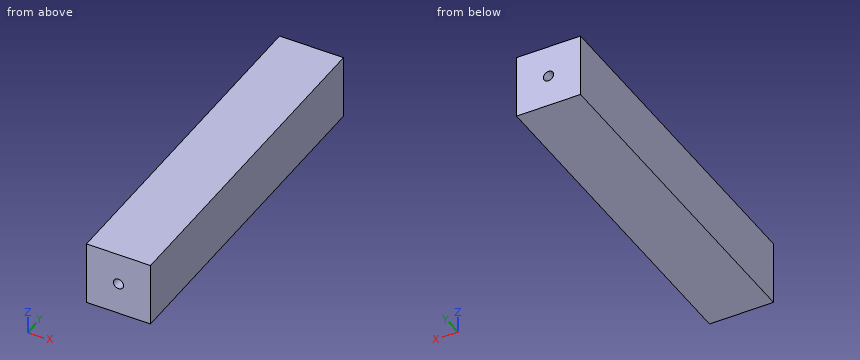
from build123d import *

# Parameters (mm, degrees)
F1_DEPTH = 250
F2_W     = 50
F2_H     = 50
F2_R     = 4
F3_DEPTH = 9.5
F4_W     = 50
F4_H     = 50
F4_R     = 4
F5_DEPTH = 9.5


with BuildPart() as f1:
    # F0 (on Front) → F1 (new body)
    with BuildSketch(Plane.XZ):
        Polygon((25, -25), (25, 0), (25, 25), (-25, 25), (-25, -25), align=None)
        Polygon((20, -20), (0, -20), (-20, -20), (-20, 20), (20, 20), align=None, mode=Mode.SUBTRACT)
    extrude(amount=F1_DEPTH)

    # F2 (on face) → F3 (join)
    with BuildSketch(Plane.XZ.offset(250)):
        Rectangle(F2_W, F2_H)
        Circle(F2_R, mode=Mode.SUBTRACT)
    extrude(amount=F3_DEPTH)

    # F4 (on face) → F5 (join)
    with BuildSketch(Plane.XZ):
        Rectangle(F4_W, F4_H)
        Circle(F4_R, mode=Mode.SUBTRACT)
    extrude(amount=-F5_DEPTH)


solid = f1.part
Here's how the part is built. I have some questions about the finished solid (model axes, mm). Give positions to 0.01 mm unless a question says otherwise; leave off trailing zeros. Order: outer loops, then holes, each group sorted by start corner. A loop starts at its lowest first (then second) coordinate and runs counter-clockwise, first axis right, second up. Notation, with made-up numbers: (-12.5, 49) -> (21.5, 49) arc R15 ccw to (21.5, 65) -> close; hole circle Ø10 at (60, -9). An arc over 180 degrees is marked (long way). Use a Markdown table: item, result. Add a question column.
Item 1: Imagine slicing it at A-A on x = 0. Please give me the cut outline in (y, z).
Item 2: I need wall thicknesses on line 1 (Z direction, x = -15, y = -199.5); line 2 (Y direction, x = 2, z = -17). Which ranges of each line are inside material? Lowest first, please.
Item 3: Imagine slicing it at B-B on z = -8. Please give me the cut outline in (x, y).
Item 4: Imagine slicing it at C-C on y = -66. Please give me the cut outline in (x, z).
Data:
| question | item | result |
|---|---|---|
| 1 | outline | (-259.5, -25) -> (9.5, -25) -> (9.5, -4) -> (0, -4) -> (0, -20) -> (-250, -20) -> (-250, -4) -> (-259.5, -4) -> close; (-259.5, 4) -> (-250, 4) -> (-250, 20) -> (0, 20) -> (0, 4) -> (9.5, 4) -> (9.5, 25) -> (-259.5, 25) -> close |
| 2 | line 1 | z = -25 to -20, 20 to 25 |
| 2 | line 2 | y = -259.5 to -250, 0 to 9.5 |
| 3 | outline | (-25, -259.5) -> (25, -259.5) -> (25, 9.5) -> (-25, 9.5) -> close; hole (-20, -250) -> (20, -250) -> (20, 0) -> (-20, 0) -> close |
| 4 | outline | (-25, -25) -> (25, -25) -> (25, 25) -> (-25, 25) -> close; hole (-20, -20) -> (20, -20) -> (20, 20) -> (-20, 20) -> close |
